from build123d import *

# Parameters (mm, degrees)
SKETCH1_W              = 69.85
SKETCH1_H              = 76.2
SKETCH1_R              = 14.2875
SKETCH1_R_2            = 2.413
BOSS_EXTRUDE1_DEPTH    = 3.175
SKETCH2_W              = 69.85
SKETCH2_H              = 3.175
BOSS_EXTRUDE2_DEPTH    = 63.5
CONVERT_SOLID1_START   = -34.925
CONVERT_SOLID1_DEPTH   = 69.85
CONVERT_SOLID1_2_DEPTH = 69.85
FILLET1_R              = 2.54
SKETCH7_R              = 2.413
CUT_EXTRUDE1_DEPTH     = 103.881758587


# Read off the part's stored shape, not the designer's step: Convert-Solid1
with BuildPart() as part:
    # Sketch1 → Boss-Extrude1 (new body)
    with BuildSketch(Plane(origin=(0, 0, 0), x_dir=(0, 0, -1), z_dir=(1, 0, 0))):
        Rectangle(SKETCH1_W, SKETCH1_H)
        with Locations((0, 6.35)):
            Circle(SKETCH1_R, mode=Mode.SUBTRACT)
        with Locations((26.67, 28.194)):
            Circle(SKETCH1_R_2, mode=Mode.SUBTRACT)
        with Locations((-26.67, -15.494)):
            Circle(SKETCH1_R_2, mode=Mode.SUBTRACT)
    extrude(amount=BOSS_EXTRUDE1_DEPTH)

    # Sketch2 → Boss-Extrude2 (add)
    with BuildSketch(Plane.ZY):
        with Locations((0, -36.5125)):
            Rectangle(SKETCH2_W, SKETCH2_H)
    extrude(amount=BOSS_EXTRUDE2_DEPTH)

    # Convert-Solid1 outline → Convert-Solid1 (cut)
    with BuildSketch(Plane.XY.offset(CONVERT_SOLID1_START)):
        with BuildLine():
            Line((3.175, -38.1), (3.175, -29.845))
            ThreePointArc((3.175, -29.845), (0.757166479, -35.682166479), (-5.08, -38.1))
            Line((-5.08, -38.1), (3.175, -38.1))
        make_face()
    extrude(amount=CONVERT_SOLID1_DEPTH, mode=Mode.SUBTRACT)

    # Convert-Solid1 2 outline → Convert-Solid1 2 (add)
    with BuildSketch(Plane.XY.offset(CONVERT_SOLID1_START)):
        with BuildLine():
            Line((0, -34.925), (0, -29.845))
            ThreePointArc((0, -29.845), (-1.487897552, -33.437102448), (-5.08, -34.925))
            Line((-5.08, -34.925), (0, -34.925))
        make_face()
    extrude(amount=CONVERT_SOLID1_2_DEPTH)

    # Fillet1
    fillet1_edges = [part.edges().sort_by_distance(p)[0] for p in [
        (1.5875, 38.1, -34.925),
        (1.5875, 38.1, 34.925),
        (-63.5, -36.5125, 34.925),
        (-63.5, -36.5125, -34.925),
    ]]
    fillet(fillet1_edges, radius=FILLET1_R)

    # Sketch7 → Cut-Extrude1 (cut, through all)
    with BuildSketch(Plane(origin=(0, -34.925, 0), x_dir=(1, 0, 0), z_dir=(0, 1, 0))):
        with Locations(Location((-50.8, 15.875, 0), (0, 0, 270))):
            Circle(SKETCH7_R)
        with Locations(Location((-20.32, 15.875, 0), (0, 0, 270))):
            Circle(SKETCH7_R)
        with Locations(Location((-50.8, -15.875, 0), (0, 0, 270))):
            Circle(SKETCH7_R)
        with Locations(Location((-20.32, -15.875, 0), (0, 0, 270))):
            Circle(SKETCH7_R)
    extrude(amount=-CUT_EXTRUDE1_DEPTH, mode=Mode.SUBTRACT)


solid = part.part
Model file for the job. Use its own axes, mm. A direction names the side the tool comes from. Give positions to 0.01 mm unless a question says otherwise; leave off trailing zeros. Order: outer loops, then holes, each group sorted by start corner. A loop starts at its lowest first (then second) coordinate and runs counter-clockwise, first axis right, second up. Notation, with made-up numbers: M -5.5,63 L 0.5,63 A20 ccw 0.5,99 Z; hole C 48.5,-0.5 d11. An arc over 180 degrees is marked long. Put each result on its own line as item: value. Start each with the question number.
(1) Pin check, flat tips, straight feed: pin 1 Ø6.5 at (y, z) = (28.194, -26.67) entering from -X; pin 2 Ø1.5 at (x, z) = (-13.5, -23.5) entering from +Y (3 decimals). Stop position of each tip, or through.
(2) Band-saw the part on C-C on z = 0. Give the cut face in (x, y) (1 decimal), then the cut area to 3 significant figures.
(3) Tool access for faces 1 (the face through (0.82, -35.62, -0.49)), 2 (the face through (0, -10, 0)): list every direction of +Z, -Z, +X, -X, +Y, -Y with a clear straight run to the whole face (end or side of a thin tool).
(4) Drill centre lines: L1, parallel to Z at x = -20, y = -36 (3 decimals); L2, parallel to Y at x = -56, z = -16 (3 decimals); L3, parallel to X at y = -28, z = 10.5 (3 decimals). Where is each one in solid material? Low to high. Write a range as [from, to].
(5) Band-saw the part on B-B on y = 6.35. Give the cut face in (x, z) (1 decimal).
(6) Band-saw the part on D-D on z = 26.67. Give the cut face in (x, y) (3 decimals), then the cut area to 3 significant figures.
(7) Pull direction Z, two halves, no side cores. Call faces 3 (the face through (-62.736, -36.49, 34.201)), 4 (the face through (-48.408, -36.49, -16.189)), 5 (the face through (2, -17, -34.925)), 6 (the face through (-34, -34.925, 0)): released by +Z, released by -Z, zero draft, split by the parting line, or undercut.
(8) Band-saw the part on A-A on x = -50.8. Give the cut face in (y, z) (3 decimals).
Results below:
1. pin 1: stops at x = 0
1. pin 2: stops at y = -34.925
2. outline: M -63.5,-38.1 L -5.1,-38.1 A8.3 ccw 3.2,-29.8 L 3.2,-7.9 L 0,-7.9 L 0,-29.8 A5.1 cw -5.1,-34.9 L -63.5,-34.9 Z; M 0,20.6 L 3.2,20.6 L 3.2,38.1 L 0,38.1 Z
2. area: 344 mm2
3. face 1: +Z, -Z, +X, -Y
3. face 2: +Z, -Z, -X, +Y
4. L1: z = [-34.925, -18.267], [-13.483, 13.483], [18.267, 34.925]
4. L2: y = [-38.1, -34.925]
4. L3: x = [0, 3.175]
5. outline: M 0,-34.9 L 3.2,-34.9 L 3.2,-14.3 L 0,-14.3 Z; M 0,14.3 L 3.2,14.3 L 3.2,34.9 L 0,34.9 Z
6. outline: M -63.5,-38.1 L -5.08,-38.1 A8.255 ccw 3.175,-29.845 L 3.175,-17.907 L 0,-17.907 L 0,-29.845 A5.08 cw -5.08,-34.925 L -63.5,-34.925 Z; M 0,-13.081 L 3.175,-13.081 L 3.175,38.1 L 0,38.1 Z
6. area: 419 mm2
7. face 3: released by +Z
7. face 4: undercut
7. face 5: released by -Z
7. face 6: zero draft
8. outline: M -38.1,-34.925 L -34.925,-34.925 L -34.925,-18.288 L -38.1,-18.288 Z; M -38.1,-13.462 L -34.925,-13.462 L -34.925,13.462 L -38.1,13.462 Z; M -38.1,18.288 L -34.925,18.288 L -34.925,34.925 L -38.1,34.925 Z
